Input: dimensioned drawing with shaded views. Units: mm. Origin: part minimum x, y, z. A direction names the side the tool comes from. Give positions to 0.01 mm unless a question says otherwise; leave off trailing zeros. Write each loop counter-clockwise with the first axis right and the second up, starting at its lowest first coordinate (ties: lowest second). Pieces come first, ordered by that corner, then holes.
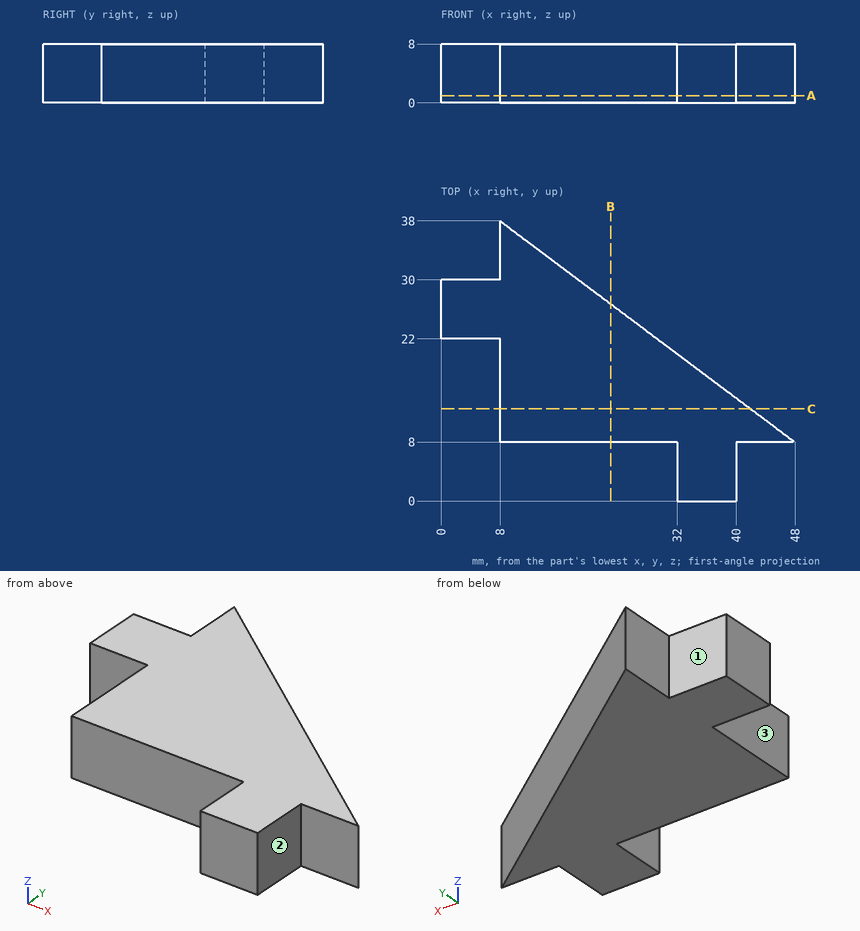
Item 1: Set-up query: the marked faces 1, 2 and 3. Return all of +Z, -Z, +X, -X, +Y, -Y with unobstructed straight access to the full face (end or side cutting, diameter ignored); none if empty.
Item 2: Section B-B (x = 23). Return loops of the section in (y, z).
Item 3: Section C-C (y = 12.5). Return loops of the section in (x, z), and give its area (3 significant figures).
Item 4: Section A-A (z = 1). Return loops of the section in (x, y), and give its area (3 significant figures).
Item 5: Ray query, line 1 (X direction, y = 2, z = 5.75); line 2 (Y direction, x = 7, z = 3); line 3 (X direction, y = 9, z = 1.25). Return the intervals inside material, ascending.
Item 6: Pin query (flat end, axial travel): pin 1 (4 mm diameter, centred on y = 3.5, z = 5.5, fed in from -X); pin 2 (2 mm diameter, centred on y = 14, z = 6, fed in from +X); pin 3 (2.5 mm diameter, centred on y = 13, z = 4.5, fed in from -X). Return the tip coordinate at first contact, or that it passes through.
Solved:
1. face 1: +Z, -Z, -X, +Y
1. face 2: +Z, -Z, +X, -Y
1. face 3: +Z, -Z, -X, -Y
2. outline: (8, 0) - (26.75, 0) - (26.75, 8) - (8, 8) - close
3. outline: (8, 0) - (42, 0) - (42, 8) - (8, 8) - close
3. area: 272 mm2
4. outline: (0, 22) - (8, 22) - (8, 8) - (32, 8) - (32, 0) - (40, 0) - (40, 8) - (48, 8) - (8, 38) - (8, 30) - (0, 30) - close
4. area: 728 mm2
5. line 1: x = 32 to 40
5. line 2: y = 22 to 30
5. line 3: x = 8 to 46.67
6. pin 1: stops at x = 32
6. pin 2: stops at x = 41.33
6. pin 3: stops at x = 8
